from build123d import *

# Parameters (mm, degrees)
SKETCH1_W           = 64
SKETCH1_H           = 32
BOSS_EXTRUDE1_DEPTH = 36
SKETCH3_R           = 6
CUT_EXTRUDE1_DEPTH  = 26
SKETCH4_R           = 6
CUT_EXTRUDE2_DEPTH  = 26
SKETCH5_W           = 16
SKETCH5_H           = 32
BOSS_EXTRUDE3_DEPTH = 9


with BuildPart() as part:
    # Sketch1 → Boss-Extrude1 (new body)
    with BuildSketch(Plane(origin=(0, 0, 0), x_dir=(1, 0, 0), z_dir=(0, 1, 0))):
        Rectangle(SKETCH1_W, SKETCH1_H)
    extrude(amount=BOSS_EXTRUDE1_DEPTH)

    # Sketch3 → Cut-Extrude1 (cut)
    with BuildSketch(Plane.XY.offset(16)):
        with BuildLine():
            Line((-32, 36), (-32, 10))
            Line((-32, 10), (-29, 10))
            ThreePointArc((-29, 10), (-27.658359214, 10.316718427), (-26.6, 11.2))
            Line((-26.6, 11.2), (-12.8, 29.6))
            ThreePointArc((-12.8, 29.6), (-7.155417528, 34.310835056), (0, 36))
            Line((0, 36), (-32, 36))
        make_face()
        with Locations((0, 20)):
            Circle(SKETCH3_R)
        with BuildLine():
            Line((32, 36), (0, 36))
            ThreePointArc((0, 36), (7.155417528, 34.310835056), (12.8, 29.6))
            Line((12.8, 29.6), (26.6, 11.2))
            ThreePointArc((26.6, 11.2), (27.658359214, 10.316718427), (29, 10))
            Line((29, 10), (32, 10))
            Line((32, 10), (32, 36))
        make_face()
    extrude(amount=-CUT_EXTRUDE1_DEPTH, mode=Mode.SUBTRACT)

    # Sketch4 → Cut-Extrude2 (cut)
    with BuildSketch(Plane.XY.offset(-10)):
        with Locations((0, 20)):
            Circle(SKETCH4_R)
    extrude(amount=-CUT_EXTRUDE2_DEPTH, mode=Mode.SUBTRACT)

    # Sketch5 → Boss-Extrude3 (add)
    with BuildSketch(Plane.XZ):
        Rectangle(SKETCH5_W, SKETCH5_H)
    extrude(amount=BOSS_EXTRUDE3_DEPTH)


solid = part.part
Geometry: final body of the model. Coordinates: model frame, mm. A direction names the side the tool comes from. Round coordinates to 2 decimals unless told otherwise and drop trailing zeros. Order: outer loops, then holes, each group sorted by start corner. A loop starts at its lowest first (then second) coordinate and runs counter-clockwise, first axis right, second up. Notation, with made-up numbers: (-11, -11.5) -> (46, -11.5) arc R28 cw to (46, 19.5) -> close; hole circle Ø10 at (84, -5). An arc over 180 degrees is marked (long way). Put each result on its own line as item: value. Start each with the question number.
Q1. First-contact query: pin 1 (1.5 mm diameter, centred on x = 30, z = 5.5, fed in from +Y); pin 2 (2.5 mm diameter, centred on y = -3.5, z = 2, fed in from +X); pin 3 (5 mm diameter, centred on x = 13, y = -3, fed in from -Z); pin 4 (12 mm diameter, centred on x = -17.5, z = 8, fed in from -Y). Flat tips, straight axial feed; report the tip coordinate or a pass-through.
Q2. Section A-A on z = -14. Return the cut outline in (x, y), and give its area (3 significant figures).
Q3. Section B-B on y = 20. Return the cut outline in (x, z), and give its area (3 significant figures).
Q4. Pull-direction query (X, two-part tool) for faces 5 (the flat face through (-20, 20, 3)), 6 (the cylindrical face through (-6, 20, 0)), 7 (the flat face through (23, 26, -10)), 8 (the flat face through (19.603, 20.529, 3.182)); classes: +X half, -X half, draft (parallel to the pull), parting line (faces both ways), or undercut.
Q5. Reachability of faces 1 (the flat face through (20, 0, 0)), 2 (the cylindrical face through (27.641, 10.325, 3.182)), 3 (the flat face through (-31, 10, 3)), 4 (the flat face through (-20, 0, 0)) from +Z, -Z, +X, -X, +Y, -Y: full face, straight path, thin tool, end or side. Return the list, or none.
Q6. Section C-C on x = 3.5. Return the cut outline in (y, z).
Q7. Section D-D on y = 13. Return the cut outline in (x, z), and give its area (3 significant figures).
Q8. Line query: probe 1 along Y at (x, z) = (0, 7); probe 2 along Z at (x, y) = (25.5, 28.5); probe 3 along Y at (x, z) = (-2.5, 3.5). Output: solid intervals per line, ascending.
Ans:
1. pin 1: stops at y = 10
1. pin 2: stops at x = 8
1. pin 3: passes through
1. pin 4: stops at y = 0
2. outline: (-32, 0) -> (-8, 0) -> (-8, -9) -> (8, -9) -> (8, 0) -> (32, 0) -> (32, 36) -> (-32, 36) -> close; hole circle Ø12 at (0, 20)
2. area: 2,330 mm2
3. outline: (-32, -16) -> (-6, -16) -> (-6, 16) -> (-20, 16) -> (-20, -10) -> (-32, -10) -> close; (6, -16) -> (32, -16) -> (32, -10) -> (20, -10) -> (20, 16) -> (6, 16) -> close
3. area: 1,040 mm2
4. face 5: -X half
4. face 6: undercut
4. face 7: draft
4. face 8: +X half
5. face 1: +Z, -Z, +X, -Y
5. face 2: +Z, +X, +Y
5. face 3: +Z, -X, +Y
5. face 4: +Z, -Z, -X, -Y
6. outline: (-9, -16) -> (15.13, -16) -> (15.13, 16) -> (-9, 16) -> close; (24.87, -16) -> (36, -16) -> (36, -10) -> (35.61, -10) -> (35.61, 16) -> (24.87, 16) -> close
7. outline: (-32, -16) -> (32, -16) -> (32, -10) -> (25.25, -10) -> (25.25, 16) -> (-25.25, 16) -> (-25.25, -10) -> (-32, -10) -> close
7. area: 1,700 mm2
8. probe 1: y = -9 to 14, 26 to 36
8. probe 2: z = -16 to -10
8. probe 3: y = -9 to 14.55, 25.45 to 35.8
